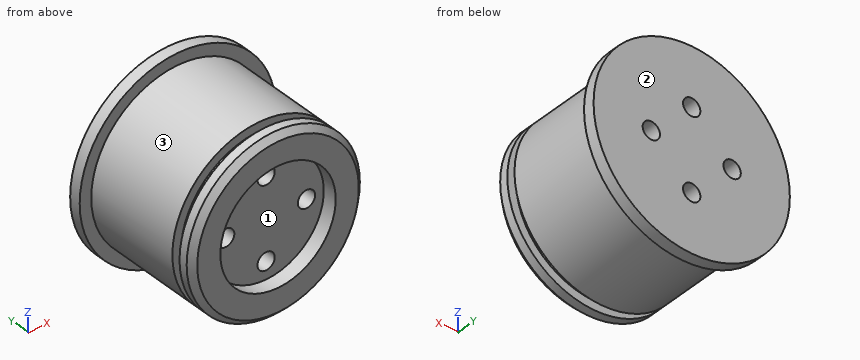
from build123d import *

# Parameters (mm, degrees)
SKETCH_1_R               = 15
EXTRUDE_1_DEPTH          = 21
SKETCH_2_R               = 10
CUT_EXTRUDE_2_DEPTH      = 2.5
SKETCH_5_R               = 15
SKETCH_5_R_2             = 13.5
CUT_EXTRUDE_5_DEPTH      = 1.5
CHAMFER_1_SIZE           = 1
SKETCH_6_R               = 17
EXTRUDE_2_DEPTH          = 2
SKETCH_4_R               = 1.5
CUT_EXTRUDE_6_DEPTH      = 32.595094556
PATTERN_CIRCULAR_1_COUNT = 4


with BuildPart() as part:
    # Эскиз1 → Бобышка-Вытянуть1 (new body)
    with BuildSketch(Plane(origin=(0, 0, 0), x_dir=(1, 0, 0), z_dir=(0, 1, 0))):
        with Locations(Location((0, 0, 0), (0, 0, 90))):
            Circle(SKETCH_1_R)
    extrude(amount=EXTRUDE_1_DEPTH)

    # Эскиз2 → Вырез-Вытянуть2 (cut)
    with BuildSketch(Plane.XZ):
        with Locations(Location((0, 0, 0), (0, 0, 270))):
            Circle(SKETCH_2_R)
    extrude(amount=-CUT_EXTRUDE_2_DEPTH, mode=Mode.SUBTRACT)

    # Эскиз5 → Вырез-Вытянуть5 (cut)
    with BuildSketch(Plane(origin=(0, 2.5, 0), x_dir=(-1, 0, 0), z_dir=(0, -1, 0))):
        with Locations(Location((0, 0, 0), (0, 0, 90))):
            Circle(SKETCH_5_R)
        with Locations(Location((0, 0, 0), (0, 0, 90))):
            Circle(SKETCH_5_R_2, mode=Mode.SUBTRACT)
    extrude(amount=-CUT_EXTRUDE_5_DEPTH, mode=Mode.SUBTRACT)

    # Фаска1
    chamfer_1_edges = [part.edges().sort_by_distance(p)[0] for p in [
        (0, 0, 15),
    ]]
    chamfer(chamfer_1_edges, length=CHAMFER_1_SIZE)

    # Эскиз6 → Бобышка-Вытянуть2 (add)
    with BuildSketch(Plane(origin=(0, 21, 0), x_dir=(1, 0, 0), z_dir=(0, 1, 0))):
        with Locations(Location((0, 0, 0), (0, 0, 270))):
            Circle(SKETCH_6_R)
    extrude(amount=EXTRUDE_2_DEPTH)

    # Эскиз4 → Вырез-Вытянуть6 (cut, through all)
    with BuildSketch(Plane.XZ.offset(-2.5)):
        with Locations(Location((0, 7, 0), (0, 0, 270))):
            Circle(SKETCH_4_R)
    cut_extrude_6 = extrude(amount=-CUT_EXTRUDE_6_DEPTH, mode=Mode.SUBTRACT)

    # Круговой массив1: Вырез-Вытянуть6 ×4 about axis
    pattern_circular_1_axis = Axis((0, 0, 0), (0, 1, 0))
    for i in range(1, PATTERN_CIRCULAR_1_COUNT):
        add(cut_extrude_6.rotate(pattern_circular_1_axis, i * 360 / PATTERN_CIRCULAR_1_COUNT), mode=Mode.SUBTRACT)


solid = part.part
Work out the finished part from the listing and answer in its coordinate system (mm). Face numbers are marked on the shaded views. Coordinates: 2 decimals unless noted, no trailing zeros. Write each loop counter-clockwise with the first axis right and the second up, starting at its lowest first coordinate (ties: lowest second). Pieces come first, ordered by that corner, then holes. Notation, with made-up numbers: M -22,82 L 37,82 A14 cw 37,104 Z; hole C -14.75,-31 d5. An arc over 180 degrees is marked long. Use one line per item in the form item = value. Start each with the question number.
1. Each of these flat-tipped pins is pushed along its axis until it touches: P1, Ø8, axis at x = -4, y = 14.5, coming from the +Z side; P2, Ø4, axis at x = 12.5, z = 12.5, coming from the -Y side; P3, Ø3, axis at x = 2.5, y = 6.5, coming from the -Z side. Where does it stop, or does it pass through?
2. The part is cut by section A-A (z = 0). Give the number of separate pieces and of enclosed holes in the cut face, plus the area to 4 significant figures.
3. Straight lines are drawn through the part: probe 1 along X at (y, z) = (1.9, 0); probe 2 along Y at (x, z) = (-5, -3.5); probe 3 along X at (y, z) = (19.25, 7). For each, find the intervals that lie inside material, in ascending order. Write a range as from..to.
4. The mould has two halves that part along Z. Classify the marked faces 1, 2 and 3: released by +Z, released by -Z, zero draft, split by the parting line, or undercut.
5. The part is cut by section C-C (y = 5.25). Give the vertices of the cut face in (x, z).
Evaluation:
q1.P1 = 15
q1.P2 = 21
q1.P3 = -14.97
q2.separate_pieces = 3
q2.enclosed_holes = 0
q2.area = 519.5 mm^2
q3.probe_1 = -15..-10, 10..15
q3.probe_2 = 2.5..23
q3.probe_3 = -13.27..-1.5, 1.5..13.27
q4.face_1 = undercut
q4.face_2 = zero draft
q4.face_3 = split by the parting line
q5.outline = C 0,0 d30; hole C -7,0 d3; hole C 0,-7 d3; hole C 0,7 d3; hole C 7,0 d3
